Read the model definition and answer for the solid it produces. Units are mm, in the model's axes. Give positions to 0.01 mm unless a question says otherwise; leave off trailing zeros. Order: outer loops, then holes, each group sorted by start corner. A loop starts at its lowest first (then second) coordinate and runs counter-clockwise, first axis right, second up. Notation, with made-up numbers: M 32,-33.75 L 66,-33.75 A21 cw 66,-20.75 Z; hole C 79.5,-26.75 d5. An arc over 180 degrees is marked long. One line per item, written item: value.
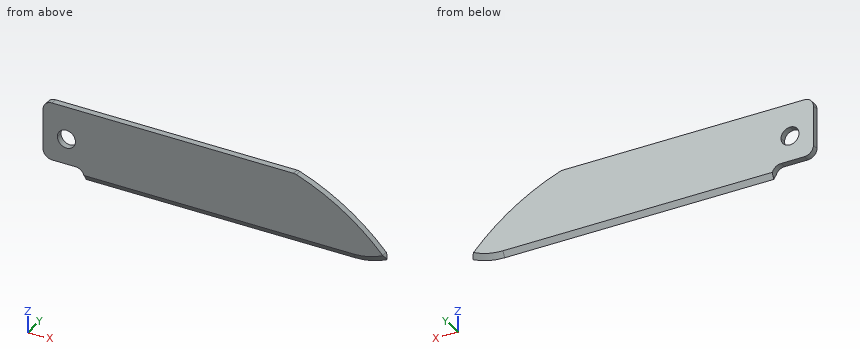
from build123d import *

# Parameters (mm, degrees)
F1_DEPTH    = 1.75
F2_F1_R     = 2.5
F2_F2_R     = 2.5
F3_T1_DEPTH = 45.6015639847
F4_T1_DEPTH = 79.2106511737
F4_T4_ANGLE = 38.8466581594
F4_T6_ANGLE = 38.8466581594


# Not quite as in the source:
# - a fillet or chamfer that OpenCascade refuses, or shapes differently, is made with other operations: its cross-section is extruded or revolved along the edge and cut away or added


with BuildPart() as f1:
    # F0 (on Front) → F1 (new body)
    with BuildSketch(Plane.XZ):
        with BuildLine():
            Line((-47.5, -6.25), (-36, -6.25))
            Line((-36, -6.25), (-36, 9.75))
            Line((-36, 9.75), (-41, 9.75))
            Line((-41, 9.75), (-41, 3.25))
            ThreePointArc((-41, 3.25), (-39.232233047, 2.517766953), (-38.5, 0.75))
            ThreePointArc((-38.5, 0.75), (-41, -1.75), (-43.5, 0.75))
            Line((-43.5, 0.75), (-47.5, 0.75))
            Line((-47.5, 0.75), (-47.5, -6.25))
        make_face()
        with BuildLine():
            Line((-36, -9.75), (47.5, -9.75))
            Line((47.5, -9.75), (47.5, -6.75))
            ThreePointArc((47.5, -6.75), (36.0462328118, 3.08520123), (22.5, 9.75))
            Line((22.5, 9.75), (-36, 9.75))
            Line((-36, 9.75), (-36, -6.25))
            Line((-36, -6.25), (-36, -9.75))
        make_face()
        with BuildLine():
            Line((-47.5, 9.75), (-47.5, 0.75))
            Line((-47.5, 0.75), (-43.5, 0.75))
            ThreePointArc((-43.5, 0.75), (-42.767766953, 2.517766953), (-41, 3.25))
            Line((-41, 3.25), (-41, 9.75))
            Line((-41, 9.75), (-47.5, 9.75))
        make_face()
    extrude(amount=F1_DEPTH)

    # F2: fillet of radius 2.5 on 5 edges, made by hand

    # F2_f1
    f2_f1_edges = [f1.edges().sort_by_distance(p)[0] for p in [
        (-36, -0.875, -6.25),
    ]]
    fillet(f2_f1_edges, radius=F2_F1_R)

    # F2_f2
    f2_f2_edges = [f1.edges().sort_by_distance(p)[0] for p in [
        (-47.5, -0.875, -6.25),
        (-47.5, -0.875, 9.75),
        (22.5, -0.875, 9.75),
        (47.5, -0.875, -6.75),
    ]]
    fillet(f2_f2_edges, radius=F2_F2_R)

    # F3: fillet of radius 20 on 1 edges, made by hand

    # F3_s2 → F3_t1 (cut)
    with BuildSketch(Plane.XZ.offset(-21.9257819924)):
        with BuildLine():
            ThreePointArc((38.7296872031, -9.75), (43.2302747659, -9.2370395799), (47.5, -7.7244711589))
            Line((47.5, -7.7244711589), (47.5, -9.75))
            Line((47.5, -9.75), (38.7296872031, -9.75))
        make_face()
    extrude(amount=F3_T1_DEPTH, mode=Mode.SUBTRACT)

    # F4: chamfer of 1 x 1.7320508076 on 4 edges, made by hand

    # F4_s2 → F4_t1 (cut)
    with BuildSketch(Plane.YZ.offset(-40.4809639706)):
        Polygon((-1.75, -8.0179491924), (-0.75, -9.75), (-1.75, -9.75), align=None)
        Polygon((0, -8.0179491924), (-1, -9.75), (0, -9.75), align=None)
    extrude(amount=F4_T1_DEPTH, mode=Mode.SUBTRACT)

    # F4_s3 → F4_t4 (revolve, cut)
    with BuildSketch(Plane(origin=(28.4995819615, 0, 22.9524885444), x_dir=(0, 1, 0), z_dir=(0.778827439, 0, 0.6272382484))):
        Polygon((0, -34.577709107), (-1, -36.3097599146), (0, -36.3097599146), align=None)
    revolve(axis=Axis((38.729687203, 0, 10.2499999998), (0, 1, 0)), revolution_arc=F4_T4_ANGLE, mode=Mode.SUBTRACT)

    # F4_s5 → F4_t6 (revolve, cut)
    with BuildSketch(Plane(origin=(28.4995819615, 0, 22.9524885444), x_dir=(0, 1, 0), z_dir=(0.778827439, 0, 0.6272382484))):
        Polygon((-1.75, -34.577709107), (-0.75, -36.3097599146), (-1.75, -36.3097599146), align=None)
    revolve(axis=Axis((38.729687203, -1.75, 10.2499999998), (0, 1, 0)), revolution_arc=F4_T6_ANGLE, mode=Mode.SUBTRACT)


solid = f1.part
1) Each of these flat-tipped pins is pushed along its axis until it touches: pin 1 Ø0.5 at (x, y) = (-42.5, -0.5) entering from -Z; pin 2 Ø1 at (x, z) = (32, 4) entering from +Y. Where does it stop, or does it pass through?
Reported:
pin 1: stops at z = -6.25
pin 2: stops at y = 0
2) Find section C-C, the plane z = -4.75. Write down the section's boundary in (x, y).
Reported:
outline: M -47.29,-1.75 L 45.61,-1.75 L 45.61,0 L -47.29,0 Z
3) Consider probe 1 along X at (y, z) = (-0.25, 2.5); probe 2 along X at (y, z) = (-0.85, 1); probe 3 along Z at (x, y) = (-18, -0.5). Determine where each line is inside the solid, lowest interval first.
Reported:
probe 1: x = -47.5 to -42.79, -39.21 to 36.92
probe 2: x = -47.5 to -43.49, -38.51 to 39.01
probe 3: z = -8.88 to 9.75
4) Find section A-A, the plane x = -39.5. Write down the section's boundary in (y, z).
Reported:
outline: M -1.75,-6.25 L 0,-6.25 L 0,-1.25 L -1.75,-1.25 Z; M -1.75,2.75 L 0,2.75 L 0,9.75 L -1.75,9.75 Z
